from build123d import *

# Parameters (mm, degrees)
SKETCH_1_R          = 1.45
EXTRUDE_1_DEPTH     = 2
EXTRUDE_2_DEPTH     = 2
SKETCH_3_R          = 6.5
CUT_EXTRUDE_1_DEPTH = 2
SKETCH_4_R          = 1.45
CUT_EXTRUDE_2_DEPTH = 1
CUT_EXTRUDE_3_DEPTH = 0.25


with BuildPart() as part:
    # Эскиз1 → Бобышка-Вытянуть1 (new body)
    with BuildSketch(Plane(origin=(0, 0, 0), x_dir=(1, 0, 0), z_dir=(0, 1, 0))):
        Polygon((35.593108597, -12.265362584), (35.593108597, 6.734637416), (32.593108597, 9.734637416), (-23.906891403, 9.734637416), (-26.906891403, 6.734637416), (-26.906891403, -12.265362584), (-23.906891403, -15.265362584), (32.593108597, -15.265362584), align=None)
        with Locations(Location((-22.906891403, -11.765362584, 0), (0, 0, 270))):
            Circle(SKETCH_1_R, mode=Mode.SUBTRACT)
        with BuildLine():
            Line((25.893108597, 8.234637416), (-15.606891403, 8.234637416))
            Line((-15.606891403, 8.234637416), (-24.906891403, 2.234637416))
            Line((-24.906891403, 2.234637416), (-24.906891403, -8.765362584))
            Line((-24.906891403, -8.765362584), (-15.008932433, -13.765362584))
            Line((-15.008932433, -13.765362584), (26.491067567, -13.765362584))
            Line((26.491067567, -13.765362584), (33.593108597, -10.265362584))
            Line((33.593108597, -10.265362584), (33.593108597, 4.734637416))
            Line((33.593108597, 4.734637416), (32.596332637, 5.187717397))
            ThreePointArc((32.596332637, 5.187717397), (32.193122866, 7.554668808), (30.144679077, 6.302105379))
            Line((30.144679077, 6.302105379), (25.893108597, 8.234637416))
        make_face(mode=Mode.SUBTRACT)
    extrude(amount=EXTRUDE_1_DEPTH)

    # Эскиз2 → Бобышка-Вытянуть2 (add)
    with BuildSketch(Plane(origin=(0, 2, 0), x_dir=(1, 0, 0), z_dir=(0, 1, 0))):
        Polygon((32.593108597, -15.265362584), (35.593108597, -12.265362584), (35.593108597, 6.734637416), (32.593108597, 9.734637416), (-23.906891403, 9.734637416), (-26.906891403, 6.734637416), (-26.906891403, -12.265362584), (-23.906891403, -15.265362584), align=None)
    extrude(amount=EXTRUDE_2_DEPTH)

    # Эскиз3 → Вырез-Вытянуть1 (cut)
    with BuildSketch(Plane(origin=(0, 4, 0), x_dir=(1, 0, 0), z_dir=(0, 1, 0))):
        with Locations(Location((-11.406891403, -2.765362584, 0), (0, 0, 270))):
            Circle(SKETCH_3_R)
    extrude(amount=-CUT_EXTRUDE_1_DEPTH, mode=Mode.SUBTRACT)

    # Эскиз4 → Вырез-Вытянуть2 (cut)
    with BuildSketch(Plane.XZ.offset(-2)):
        with Locations(Location((31.593108597, -6.234637416, 0), (0, 0, 270))):
            Circle(SKETCH_4_R)
        with Locations(Location((-22.906891403, 11.765362584, 0), (0, 0, 270))):
            Circle(SKETCH_4_R)
    extrude(amount=-CUT_EXTRUDE_2_DEPTH, mode=Mode.SUBTRACT)

    # Эскиз5 → Вырез-Вытянуть3 (cut)
    with BuildSketch(Plane(origin=(0, 4, 0), x_dir=(1, 0, 0), z_dir=(0, 1, 0))):
        with BuildLine():
            Line((8.980608597, -2.500998747), (8.980608597, -9.758351134))
            ThreePointArc((8.980608597, -9.758351134), (9.244212494, -10.394747237), (9.880608597, -10.658351134))
            Line((9.880608597, -10.658351134), (10.330608597, -10.658351134))
            ThreePointArc((10.330608597, -10.658351134), (10.9670047, -10.394747237), (11.230608597, -9.758351134))
            Line((11.230608597, -9.758351134), (11.230608597, -5.827862584))
            ThreePointArc((11.230608597, -5.827862584), (11.395361032, -5.43011502), (11.793108597, -5.265362584))
            Line((11.793108597, -5.265362584), (15.393108597, -5.265362584))
            ThreePointArc((15.393108597, -5.265362584), (15.790856161, -5.43011502), (15.955608597, -5.827862584))
            Line((15.955608597, -5.827862584), (15.955608597, -9.758351134))
            ThreePointArc((15.955608597, -9.758351134), (16.219212494, -10.394747237), (16.855608597, -10.658351134))
            Line((16.855608597, -10.658351134), (17.305608597, -10.658351134))
            ThreePointArc((17.305608597, -10.658351134), (17.9420047, -10.394747237), (18.205608597, -9.758351134))
            Line((18.205608597, -9.758351134), (18.205608597, -2.500998747))
            ThreePointArc((18.205608597, -2.500998747), (18.530385824, -1.991200617), (19.129676627, -2.070098747))
            Line((19.129676627, -2.070098747), (20.756009257, -3.434753858))
            ThreePointArc((20.756009257, -3.434753858), (21.166602393, -3.564213376), (21.548477287, -3.365421889))
            Line((21.548477287, -3.365421889), (22.153040559, -2.644931438))
            ThreePointArc((22.153040559, -2.644931438), (22.282500077, -2.234338302), (22.08370859, -1.852463408))
            Line((22.08370859, -1.852463408), (18.519278144, 1.138448864))
            ThreePointArc((18.519278144, 1.138448864), (18.180914744, 1.333803064), (17.796142083, 1.401648866))
            Line((17.796142083, 1.401648866), (16.855608597, 1.401648866))
            ThreePointArc((16.855608597, 1.401648866), (16.219212494, 1.138044969), (15.955608597, 0.501648866))
            Line((15.955608597, 0.501648866), (15.955608597, -2.535851134))
            ThreePointArc((15.955608597, -2.535851134), (15.790856161, -2.933598699), (15.393108597, -3.098351134))
            Line((15.393108597, -3.098351134), (11.793108597, -3.098351134))
            ThreePointArc((11.793108597, -3.098351134), (11.395361032, -2.933598699), (11.230608597, -2.535851134))
            Line((11.230608597, -2.535851134), (11.230608597, 0.501648866))
            ThreePointArc((11.230608597, 0.501648866), (10.9670047, 1.138044969), (10.330608597, 1.401648866))
            Line((10.330608597, 1.401648866), (9.39007511, 1.401648866))
            ThreePointArc((9.39007511, 1.401648866), (9.005302449, 1.333803064), (8.666939049, 1.138448864))
            Line((8.666939049, 1.138448864), (5.102508603, -1.852463408))
            ThreePointArc((5.102508603, -1.852463408), (4.903717116, -2.234338302), (5.033176634, -2.644931438))
            Line((5.033176634, -2.644931438), (5.637739906, -3.365421889))
            ThreePointArc((5.637739906, -3.365421889), (6.0196148, -3.564213376), (6.430207936, -3.434753858))
            Line((6.430207936, -3.434753858), (8.056540566, -2.070098747))
            ThreePointArc((8.056540566, -2.070098747), (8.655831369, -1.991200617), (8.980608597, -2.500998747))
        make_face()
        with BuildLine():
            Line((13.593108597, 4.226315266), (10.66501019, 6.683281559))
            ThreePointArc((10.66501019, 6.683281559), (10.172298427, 6.838632981), (9.714048554, 6.600083196))
            Line((9.714048554, 6.600083196), (9.08803108, 5.854024623))
            ThreePointArc((9.08803108, 5.854024623), (8.932679658, 5.36131286), (9.171229443, 4.903062987))
            Line((9.171229443, 4.903062987), (13.014599748, 1.678092382))
            ThreePointArc((13.014599748, 1.678092382), (13.593108597, 1.467532381), (14.171617445, 1.678092382))
            Line((14.171617445, 1.678092382), (18.01498775, 4.903062987))
            ThreePointArc((18.01498775, 4.903062987), (18.253537535, 5.36131286), (18.098186113, 5.854024623))
            Line((18.098186113, 5.854024623), (17.472168639, 6.600083196))
            ThreePointArc((17.472168639, 6.600083196), (17.013918766, 6.838632981), (16.521207003, 6.683281559))
            Line((16.521207003, 6.683281559), (13.593108597, 4.226315266))
        make_face()
    extrude(amount=-CUT_EXTRUDE_3_DEPTH, mode=Mode.SUBTRACT)


solid = part.part
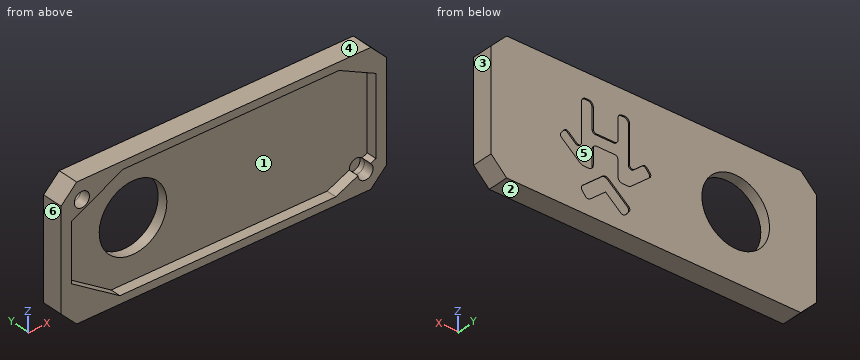
Could you check a few things on this model? Use its own coordinates, in mm. Face numbers are marked on the shaded views. A direction names the side the tool comes from. Give positions to 0.01 mm unless a question says otherwise; leave off trailing zeros. Write each loop counter-clockwise with the first axis right and the second up, starting at its lowest first coordinate (ties: lowest second). Pieces come first, ordered by that corner, then holes. Notation, with made-up numbers: (62, -21) - (109, -21) arc R25 cw to (109, 17) - close; hole circle Ø9 at (69.25, 85.5). An arc over 180 degrees is marked (long way). Use CSV: the item, a comma, the result in double quotes. Start each with the question number.
Item 1: I want a section at C-C, the plane x = -13. Please give me the cut outline in (y, z).
Item 2: If we mould it in two halves opening along X, with no side actions, what happens to the marked faces 3, 4, 5 and 6? For each: pulls with the +X half, pulls with the -X half, needs draft (parallel to the pull), parting line crosses it, or undercut.
Item 3: I want a section at D-D, the plane x = 7.5. Please give me the cut outline in (y, z).
Item 4: For the marked faces 1 and 2, which set-ups out of +Z, -Z, +X, -X, +Y, -Y let a thin tool reach every point of the face, with its end or its side?
Item 5: I want a section at B-B, the plane z = 7. Please give me the cut outline in (x, y).
Item 6: I want a section at A-A, the plane x = -1.5. Please give me the cut outline in (y, z), then the cut area to 3 significant figures.
Item 7: If I drill on line 1 along Z through (x, y) = (-11, 3); line 2 along X through (y, z) = (0.7, 4); line 3 along Z through (x, y) = (5, 0.2), over which ranges is the centre line in solid material (lowest first)?
Item 8: I'm going to push flat-ended pins straight in: pin 1 (1.7 mm diameter, centred on x = -22.91, z = 11.77, fed in from -Y); pin 2 (2 mm diameter, centred on x = -14.5, z = 6.5, fed in from -Y); pin 3 (11 mm diameter, centred on x = -0.5, z = 0.5, fed in from -Y). Where does each tip first touch, or does it pass through?
Findings:
1,outline,"(0, -9.73) - (4, -9.73) - (4, -3.54) - (2, -3.54) - (2, -8.23) - (0, -8.23) - close; (0, 13.77) - (2, 13.77) - (2, 9.07) - (4, 9.07) - (4, 15.27) - (0, 15.27) - close"
2,face 3,"pulls with the +X half"
2,face 4,"needs draft"
2,face 5,"undercut"
2,face 6,"pulls with the -X half"
3,outline,"(0, -9.73) - (4, -9.73) - (4, -0.16) - (3.75, -0.16) - (3.75, 2.54) - (4, 2.54) - (4, 15.27) - (0, 15.27) - (0, 13.77) - (2, 13.77) - (2, -8.23) - (0, -8.23) - close"
4,face 1,"-Y"
4,face 2,"-Z, +X, -X, +Y, -Y"
5,outline,"(-26.91, 0) - (-24.91, 0) - (-24.91, 2) - (-16.34, 2) - (-16.34, 4) - (-26.91, 4) - close; (-6.48, 2) - (33.59, 2) - (33.59, 0) - (35.59, 0) - (35.59, 4) - (18.21, 4) - (18.21, 3.75) - (15.96, 3.75) - (15.96, 4) - (11.23, 4) - (11.23, 3.75) - (8.98, 3.75) - (8.98, 4) - (-6.48, 4) - close"
6,outline,"(0, -9.73) - (4, -9.73) - (4, 15.27) - (0, 15.27) - (0, 13.77) - (2, 13.77) - (2, -8.23) - (0, -8.23) - close"
6,area,"56.0 mm2"
7,line 1,"z = -9.73 to -3.72, 9.25 to 15.27"
7,line 2,"x = -26.91 to -24.91, 33.59 to 35.59"
7,line 3,"z = -9.73 to -8.23, 13.77 to 15.27"
8,pin 1,"stops at y = 3"
8,pin 2,"passes through"
8,pin 3,"stops at y = 2"
